Geometry: see drawing. Coordinates: mm, zero at the bounding-box minimum. A direction names the side the tool comes from. Round coordinates to 2 decimals unless told otherwise and drop trailing zeros. Loops run counter-clockwise (first coordinate to the right, second up) from the corner with the lowest first, then second, coordinate; pieces in that order, holes last. Notation, with made-up numbers: (71, 57) - (128, 57) arc R33 ccw to (128, 86) - close; hole circle Ø9 at (15.25, 81). An arc over 180 degrees is marked (long way). Return JSON: item names as keys, results as strings. Group by question number.
1. Section C-C on z = 58.5. Return loops of the section in (x, y).
2. Section A-A on y = 12.5. Return loops of the section in (x, z).
3. Section D-D on z = 12.5. Return loops of the section in (x, y).
4. Set-up query: the marked faces 1, 2 and 3. Return all of +Z, -Z, +X, -X, +Y, -Y with unobstructed straight access to the full face (end or side cutting, diameter ignored); none if empty.
5. First-contact query: pin 1 Ø10 at (x, y) = (17, 19) entering from +Z; pin 2 Ø2 at (y, z) = (3.5, 29) entering from -X; pin 3 Ø1.5 at (x, z) = (13, 34) entering from -Y; pin 4 Ø3 at (y, z) = (3, 63) entering from -X. Flat tips, straight axial feed; report the tip coordinate or a pass-through.
6. Material intervals for probe 1 along Z at (x, y) = (9.5, 9.5); probe 2 along X at (y, z) = (12.5, 19.5); probe 3 along Z at (x, y) = (9.75, 14.25), sorted ascending.
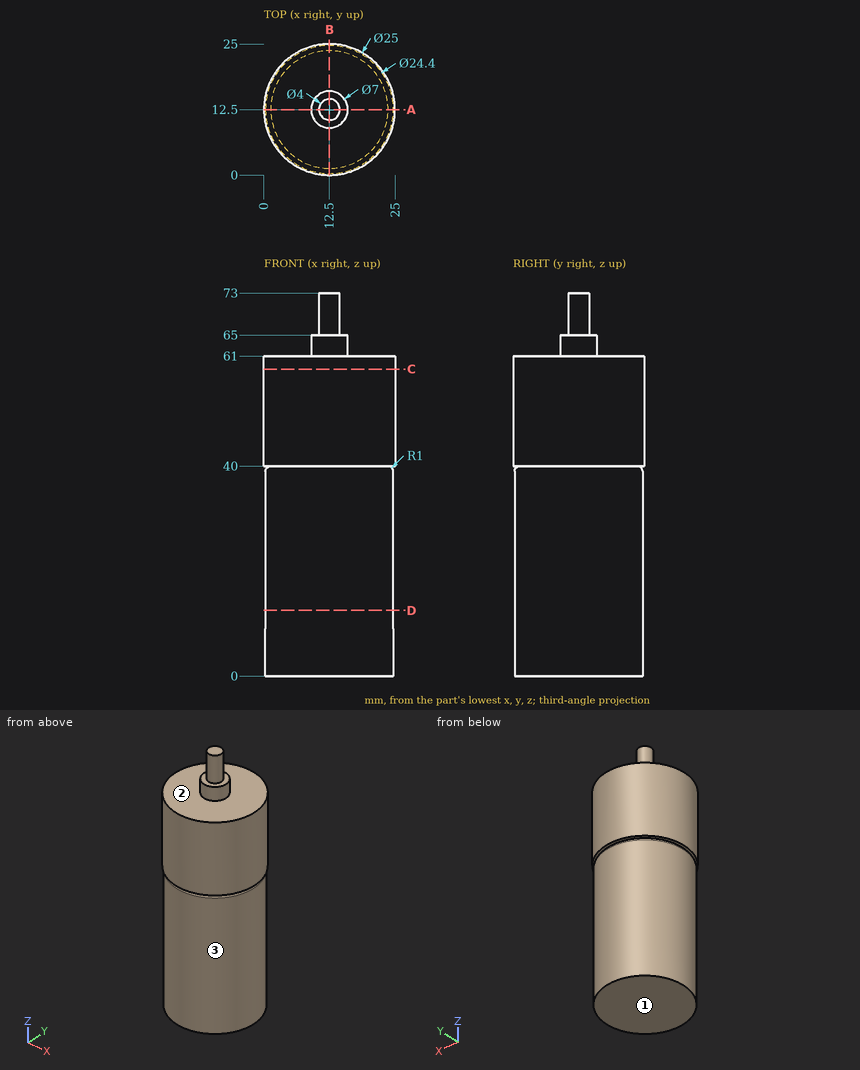
Taken from the geometry:
{
 "1": {"outline": "circle Ø25 at (12.5, 12.5)"},
 "2": {"outline": "(0, 40) - (1.3, 40) arc R1 ccw to (0.3, 39) - (0.3, 0) - (24.7, 0) - (24.7, 39) arc R1 ccw to (23.7, 40) - (25, 40) - (25, 61) - (16, 61) - (16, 65) - (14.5, 65) - (14.5, 73) - (10.5, 73) - (10.5, 65) - (9, 65) - (9, 61) - (0, 61) - close"},
 "3": {"outline": "circle Ø24.4 at (12.5, 12.5)"},
 "4": {"face 1": "-Z, +X, -X, +Y, -Y", "face 2": "+Z", "face 3": "-Z"},
 "5": {"pin 1": "z = 65", "pin 2": "x = 3.29", "pin 3": "y = 0.3", "pin 4": "through"},
 "6": {"probe 1": "0 to 61", "probe 2": "0.3 to 24.7", "probe 3": "0 to 65"}
}
